CAD build for the part. Positions are in the model's coordinates, mm. A direction names the side the tool comes from. Round coordinates to 2 decimals unless told otherwise and drop trailing zeros. Loops run counter-clockwise (first coordinate to the right, second up) from the corner with the lowest first, then second, coordinate; pieces in that order, holes last. Notation, with made-up numbers: M -28,20.5 L 21,20.5 A11 ccw 21,31.5 Z; hole C -14.5,49.5 d2. An arc over 180 degrees is marked long. Use a Markdown table: item, result. Add a question column.
(1) Wall check: L1, parallel to Y at x = 6, z = 20; L2, parallel to Z at x = 6.6, y = -3.75; L3, parallel to Y at x = 6.45, z = 34. Give the ranges that are in metal, low to high.
(2) Band-saw the part on A-A, the plane y = 3.75. Write the cut outline in (x, z).
(3) Two-plate mould, pull along Z, no slides. Class faces 4 (the face through (6.29, -2.78, 21.27)), 5 (the face through (6.29, -0.07, 35.6)), 6 (the face through (7, 0, 40)), 7 (the face through (11, 0, 0)): released by +Z, released by -Z, zero draft, split by the parting line, or undercut.
(4) Flat gauge pins, fed straight in: P1, Ø2.5, axis at y = 3.75, z = 20, coming from the +X side; P2, Ø1.5, axis at y = 1, z = 14.5, coming from the +X side; P3, Ø3.5, axis at y = -3.75, z = 20, coming from the +X side; P4, Ø2, axis at x = 14, y = 5.5, coming from the +Z side. Where does each tip first touch, or does it go through?
(5) Which spindle directions (+Z, -Z, +X, -X, +Y, -Y) get a long thin tool onto all of the face, cutting with end or side? Do faces 1 (the face through (8, -7.5, 15)), 2 (the face through (9, 3.8, 2.9)), 3 (the face through (8.5, 0, 23)). Say none if no direction does.
(6) Band-saw the part on D-D, the plane z = 20. Write the cut outline in (x, y), and give its area (3 significant figures).
(7) Band-saw the part on B-B, the plane z = 34. Write the cut outline in (x, y).
(8) Band-saw the part on C-C, the plane x = 6.5. Write the cut outline in (y, z).
Autodesk Inventor part; units mm, degrees
ref_plane "YZ Plane" through (0, 0, 0) normal (1, 0, 0) x (0, 1, 0)
ref_plane "XZ Plane" through (0, 0, 0) normal (0, 1, 0) x (-1, 0, 0)
ref_plane "XY Plane" through (0, 0, 0) normal (0, 0, 1) x (1, 0, 0)
ref_plane "Work Plane1" through (0, 0, 0) normal (0, 0, 1) x (1, 0, 0)
sketch "Sketch1" plane through (0, 0, 0) normal (0, 0, 1) x (1, 0, 0)
  circle A0 centre (0, 0) radius 20 construction
  circle A1 centre (10.45, 12.5) radius 1.75 construction
  circle A2 centre (10.45, -12.5) radius 1.75 construction
  circle A3 centre (-10.45, 12.5) radius 1.75 construction
  circle A4 centre (-10.45, -12.5) radius 1.75 construction
  line L0 (-6.5984, 12.21) -> (-6.5984, 15.25) construction
  line L1 (-6.5984, 15.25) -> (6.6016, 15.25) construction
  line L2 (6.6016, 15.25) -> (6.6016, 12.21) construction
  line L3 (6.6016, 12.21) -> (-6.5984, 12.21) construction
  line L4 (6.6016, -12.21) -> (6.6016, -15.25) construction
  line L5 (6.6016, -15.25) -> (-6.5984, -15.25) construction
  line L6 (-6.5984, -15.25) -> (-6.5984, -12.21) construction
  line L7 (-6.5984, -12.21) -> (6.6016, -12.21) construction
  line L8 (5.5, 7.5) -> (5.5, -7.5)
  line L9 (5.5, -7.5) -> (8.5, -7.5)
  line L10 (8.5, -7.5) -> (8.5, 7.5)
  line L11 (8.5, 7.5) -> (5.5, 7.5)
  line L12 (5.5, 7.5) -> (8.5, -7.5) construction
  line L13 (5.5, -7.5) -> (8.5, 7.5) construction
  line L14 (0, 0) -> (7, 0) construction
  point P0 (0, 0)
  dimension "d0" = 7
  dimension "d1" = 3
  dimension "d2" = 15
extrude "Extrusion1" add sketch "Sketch1" along normal blind 40
sketch "Sketch2" plane through (0, 0, 0) normal (0, 0, -1) x (-1, 0, 0)
  line L0 (-5.5, -7.5) -> (-8.5, -7.5)
  line L1 (-8.5, 7.5) -> (-5.5, 7.5)
  line L2 (-8.5, -7.5) -> (-8.5, 7.5)
  line L3 (-8.5, 7.5) -> (-16.5, 7.5)
  line L4 (-16.5, 7.5) -> (-16.5, -7.5)
  line L5 (-16.5, -7.5) -> (-8.5, -7.5)
  point P0 (0, 0)
  dimension "d5" = 8
extrude "Extrusion2" add sketch "Sketch2" against normal blind 2
sketch "Sketch3" plane through (0, 0, 2) normal (0, 0, 1) x (1, 0, 0)
  line L0 (16.5, -7.5) -> (16.5, 7.5) construction
  line L1 (16.5, 7.5) -> (8.5, 7.5) construction
  line L2 (8.5, -7.5) -> (8.5, 7.5) construction
  line L3 (8.5, -7.5) -> (16.5, -7.5) construction
  point P0 (0, 0)
  point P1 (12.5, 3.75)
  point P2 (12.5, -3.75)
  dimension "d9" = 3.75
  dimension "d10" = 4
  dimension "d11" = 3.75
  dimension "d12" = 4
hole "Hole1" at (12.5, 3.75, 2) at (12.5, -3.75, 2) direction (0, 0, -1) diameter 3.2 end through all
sketch "Sketch4" plane through (8.5, -7.5, 40) normal (1, 0, 0) x (0, 0, -1)
  line L0 (0, 0) -> (0, 15)
  line L1 (38, 0) -> (0, 0)
  line L2 (38, 15) -> (0, 15)
  point P0 (40, 7.5)
  point P1 (6, 7.5)
  point P2 (20, 3.75)
  point P3 (20, 11.25)
  dimension "d20" = 20
  dimension "d21" = 20
  dimension "d22" = 3.75
  dimension "d23" = 3.75
  dimension "d24" = 7.5
  dimension "d25" = 6
hole "Hole2" at (8.5, 0, 34) at (8.5, -3.75, 20) at (8.5, 3.75, 20) direction (-1, 0, 0) diameter 3.2 end through all countersink diameter 6 countersink angle 90
sketch "Sketch5" plane through (0, 0, 2) normal (0, 0, 1) x (1, 0, 0)
  circle A0 centre (12.5, 3.75) radius 1.6
  circle A1 centre (12.5, -3.75) radius 1.6
  circle A2 centre (12.5, 3.75) radius 3.5
  circle A3 centre (12.5, -3.75) radius 3.5
  point P0 (0, 0)
  dimension "d37" = 7
  dimension "d38" = 7
extrude "Extrusion3" cut sketch "Sketch5" against normal blind 0.1
fillet "Fillet2" radius 5 1 edges at (8.5, 0, 2)
properties part number "colorSensorHolder2"
Return value:
| question | item | result |
|---|---|---|
| 1 | L1 | -7.5 to -5.35, -2.15 to 2.15, 5.35 to 7.5 |
| 1 | L2 | 0 to 18.4, 21.6 to 40 |
| 1 | L3 | -7.5 to -1.6, 1.6 to 7.5 |
| 2 | outline | M 5.5,0 L 10.9,0 L 10.9,1.9 L 9,1.9 L 9,4.82 A5 cw 8.5,7 L 8.5,17 L 7.1,18.4 L 5.5,18.4 Z; M 5.5,21.6 L 7.1,21.6 L 8.5,23 L 8.5,40 L 5.5,40 Z; M 14.1,0 L 16.5,0 L 16.5,2 L 16,2 L 16,1.9 L 14.1,1.9 Z |
| 3 | face 4 | undercut |
| 3 | face 5 | undercut |
| 3 | face 6 | released by +Z |
| 3 | face 7 | released by -Z |
| 4 | P1 | through |
| 4 | P2 | x = 8.5 |
| 4 | P3 | x = 7.25 |
| 4 | P4 | z = 1.9 |
| 5 | face 1 | +Z, -Z, +X, -X, -Y |
| 5 | face 2 | +Z |
| 5 | face 3 | +Z, +X, +Y, -Y |
| 6 | outline | M 5.5,-7.5 L 8.5,-7.5 L 8.5,-6.75 L 7.1,-5.35 L 5.5,-5.35 Z; M 5.5,-2.15 L 7.1,-2.15 L 8.5,-0.75 L 8.5,0.75 L 7.1,2.15 L 5.5,2.15 Z; M 5.5,5.35 L 7.1,5.35 L 8.5,6.75 L 8.5,7.5 L 5.5,7.5 Z |
| 6 | area | 21.9 mm^2 |
| 7 | outline | M 5.5,-7.5 L 8.5,-7.5 L 8.5,-3 L 7.1,-1.6 L 5.5,-1.6 Z; M 5.5,1.6 L 7.1,1.6 L 8.5,3 L 8.5,7.5 L 5.5,7.5 Z |
| 8 | outline | M -7.5,0 L 7.5,0 L 7.5,40 L -7.5,40 Z; hole C -3.75,20 d3.2; hole C 0,34 d3.2; hole C 3.75,20 d3.2 |
